Build history of the part. All positions in model axes, mm. A direction names the side the tool comes from. Round coordinates to 2 decimals unless told otherwise and drop trailing zeros. Write each loop counter-clockwise with the first axis right and the second up, starting at its lowest first coordinate (ties: lowest second). Pieces come first, ordered by that corner, then holes. Notation, with made-up numbers: (67, 62) -> (115, 62) arc R23 ccw to (115, 87) -> close; hole circle Ø7 at (26.25, 85.5). An arc over 180 degrees is marked (long way). Return JSON: item names as keys, results as strings.
from build123d import *

# Parameters (mm, degrees)
SKETCH_1_W               = 105
SKETCH_1_H               = 115
SKETCH_1_R               = 3.5
SKETCH_1_R_2             = 1.55
EXTRUDE_1_DEPTH          = 4
SKETCH_2_R               = 45
SKETCH_2_R_2             = 32.5
CUT_EXTRUDE_1_DEPTH      = 2
SKETCH_3_R               = 10.05
SKETCH_3_R_2             = 1.7
CUT_EXTRUDE_2_DEPTH      = 1
CUT_EXTRUDE_5_DEPTH      = 20
CUT_EXTRUDE_5_DEPTH_BACK = 20
SKETCH_4_R               = 1.7


with BuildPart() as part:
    # 草图1 → 凸台-拉伸1 (new body)
    with BuildSketch(Plane(origin=(0, 0, 0), x_dir=(1, 0, 0), z_dir=(0, 1, 0))):
        Rectangle(SKETCH_1_W, SKETCH_1_H)
        with Locations(Location((0, 0, 0), (0, 0, 270))):
            Circle(SKETCH_1_R, mode=Mode.SUBTRACT)
        with Locations(Location((45, 49, 0), (0, 0, 270))):
            Circle(SKETCH_1_R_2, mode=Mode.SUBTRACT)
        with Locations(Location((45, -49, 0), (0, 0, 90))):
            Circle(SKETCH_1_R_2, mode=Mode.SUBTRACT)
        with Locations(Location((-45, -49, 0), (0, 0, 270))):
            Circle(SKETCH_1_R_2, mode=Mode.SUBTRACT)
        with Locations(Location((-45, 49, 0), (0, 0, 90))):
            Circle(SKETCH_1_R_2, mode=Mode.SUBTRACT)
        with Locations(Location((-15, -49, 0), (0, 0, 270))):
            Circle(SKETCH_1_R_2, mode=Mode.SUBTRACT)
        with Locations(Location((15, -49, 0), (0, 0, 90))):
            Circle(SKETCH_1_R_2, mode=Mode.SUBTRACT)
        with Locations(Location((15, 49, 0), (0, 0, 270))):
            Circle(SKETCH_1_R_2, mode=Mode.SUBTRACT)
        with Locations(Location((-15, 49, 0), (0, 0, 90))):
            Circle(SKETCH_1_R_2, mode=Mode.SUBTRACT)
        with Locations(Location((30, 49, 0), (0, 0, 270))):
            Circle(SKETCH_1_R_2, mode=Mode.SUBTRACT)
        with Locations(Location((-30, 49, 0), (0, 0, 270))):
            Circle(SKETCH_1_R_2, mode=Mode.SUBTRACT)
        with Locations(Location((-30, -49, 0), (0, 0, 270))):
            Circle(SKETCH_1_R_2, mode=Mode.SUBTRACT)
        with Locations(Location((30, -49, 0), (0, 0, 270))):
            Circle(SKETCH_1_R_2, mode=Mode.SUBTRACT)
    extrude(amount=EXTRUDE_1_DEPTH)

    # 草图2 → 切除-拉伸1 (cut)
    with BuildSketch(Plane(origin=(0, 4, 0), x_dir=(1, 0, 0), z_dir=(0, 1, 0))):
        with Locations(Location((0, 0, 0), (0, 0, 270))):
            Circle(SKETCH_2_R)
        with Locations(Location((0, 0, 0), (0, 0, 270))):
            Circle(SKETCH_2_R_2, mode=Mode.SUBTRACT)
    extrude(amount=-CUT_EXTRUDE_1_DEPTH, mode=Mode.SUBTRACT)

    # 草图3 → 切除-拉伸2 (cut)
    with BuildSketch(Plane(origin=(0, 4, 0), x_dir=(1, 0, 0), z_dir=(0, 1, 0))):
        with Locations(Location((0, 0, 0), (0, 0, 270))):
            Circle(SKETCH_3_R)
        with Locations(Location((0, 7, 0), (0, 0, 270))):
            Circle(SKETCH_3_R_2, mode=Mode.SUBTRACT)
        with Locations(Location((7, 0, 0), (0, 0, 270))):
            Circle(SKETCH_3_R_2, mode=Mode.SUBTRACT)
        with Locations(Location((0, -7, 0), (0, 0, 270))):
            Circle(SKETCH_3_R_2, mode=Mode.SUBTRACT)
        with Locations(Location((-7, 0, 0), (0, 0, 270))):
            Circle(SKETCH_3_R_2, mode=Mode.SUBTRACT)
    extrude(amount=-CUT_EXTRUDE_2_DEPTH, mode=Mode.SUBTRACT)

    # 草图4 → 切除-拉伸5 (cut, two sides: drawn at the far end of the back side and taken through both)
    with BuildSketch(Plane(origin=(0, 3, 0), x_dir=(1, 0, 0), z_dir=(0, 1, 0)).offset(-CUT_EXTRUDE_5_DEPTH_BACK)):
        with Locations(Location((7, 0, 0), (0, 0, 90))):
            Circle(SKETCH_4_R)
        with Locations(Location((0, 7, 0), (0, 0, 90))):
            Circle(SKETCH_4_R)
        with Locations(Location((0, -7, 0), (0, 0, 90))):
            Circle(SKETCH_4_R)
        with Locations(Location((-7, 0, 0), (0, 0, 90))):
            Circle(SKETCH_4_R)
    extrude(amount=CUT_EXTRUDE_5_DEPTH + CUT_EXTRUDE_5_DEPTH_BACK, mode=Mode.SUBTRACT)


solid = part.part
Q1. Two-plate mould, pull along X, no slides. Class faces 1 (the flat face through (-52.5, 2, 1)), 2 (the cylindrical face through (-5.34, 1.48, 0.37)), 3 (the flat face through (-1, 2, 57.5)): +X half, -X half, draft (parallel to the pull), parting line (faces both ways), or undercut.
Verdict:
{"face 1": "-X half", "face 2": "undercut", "face 3": "draft"}
Q2. Wall check: L1, parallel to Z at x = 0, y = 1.15; L2, parallel to Z at x = -13, y = 3.15; L3, parallel to Z at x = 7, y = 1. Give the ranges that are in metal, low to high.
Verdict:
{"L1": "z = -57.5 to -8.7, -5.3 to -3.5, 3.5 to 5.3, 8.7 to 57.5", "L2": "z = -57.5 to -43.08, -29.79 to 29.79, 43.08 to 57.5", "L3": "z = -57.5 to -1.7, 1.7 to 57.5"}
Q3. Pin check, flat tip, straight feed: pin 1 Ø10 at (x, z) = (-4, -2.5) entering from +Y. Stop position of the tip, or through.
Verdict:
{"pin 1": "stops at y = 3"}
Q4. 3-axis set-ups, long thin cutter, end or side, ignore diameter. For faces 4 (the flat face through (0, 3, 4)), 5 (the cylindrical face through (-45.594, 1.972, 50.432)): which of +Z, -Z, +X, -X, +Y, -Y reach the whole face in a straight line?
Verdict:
{"face 4": "+Y", "face 5": "+Y, -Y"}
Q5. Saw through at D-D on x = -7. List the corners of the cut face in (y, z).
Verdict:
{"outline": "(0, -57.5) -> (4, -57.5) -> (4, -44.45) -> (2, -44.45) -> (2, -31.74) -> (4, -31.74) -> (4, -7.21) -> (3, -7.21) -> (3, -1.7) -> (0, -1.7) -> close; (0, 1.7) -> (3, 1.7) -> (3, 7.21) -> (4, 7.21) -> (4, 31.74) -> (2, 31.74) -> (2, 44.45) -> (4, 44.45) -> (4, 57.5) -> (0, 57.5) -> close"}
Q6. Saw through at B-B on x = 15. List the corners of the cut face in (y, z).
Verdict:
{"outline": "(0, -57.5) -> (4, -57.5) -> (4, -50.55) -> (0, -50.55) -> close; (0, -47.45) -> (4, -47.45) -> (4, -42.43) -> (2, -42.43) -> (2, -28.83) -> (4, -28.83) -> (4, 28.83) -> (2, 28.83) -> (2, 42.43) -> (4, 42.43) -> (4, 47.45) -> (0, 47.45) -> close; (0, 50.55) -> (4, 50.55) -> (4, 57.5) -> (0, 57.5) -> close"}
Q7. Saw through at A-A on z = -7. List the corners of the cut face in (x, y).
Verdict:
{"outline": "(-52.5, 0) -> (-1.7, 0) -> (-1.7, 3) -> (-7.21, 3) -> (-7.21, 4) -> (-31.74, 4) -> (-31.74, 2) -> (-44.45, 2) -> (-44.45, 4) -> (-52.5, 4) -> close; (1.7, 0) -> (52.5, 0) -> (52.5, 4) -> (44.45, 4) -> (44.45, 2) -> (31.74, 2) -> (31.74, 4) -> (7.21, 4) -> (7.21, 3) -> (1.7, 3) -> close"}
Q8. Saw through at C-C on z = 43.5. List the corners of the cut face in (x, y).
Verdict:
{"outline": "(-52.5, 0) -> (52.5, 0) -> (52.5, 4) -> (11.52, 4) -> (11.52, 2) -> (-11.52, 2) -> (-11.52, 4) -> (-52.5, 4) -> close"}
